Read the model definition and answer for the solid it produces. Units are mm, in the model's axes. Face numbers are marked on the shaded views. A direction names the side the tool comes from. Coordinates: 2 decimals unless noted, no trailing zeros. Write each loop counter-clockwise with the first axis right and the second up, starting at its lowest first coordinate (ties: lowest second). Pieces come first, ordered by that corner, then holes. Notation, with made-up numbers: (-5.5, -6) -> (41.5, -6) arc R10 ccw to (41.5, 13) -> close; hole circle Ø10 at (21, -19). An arc over 180 degrees is marked (long way). Use CSV: the item, a comma, the result in double quotes.
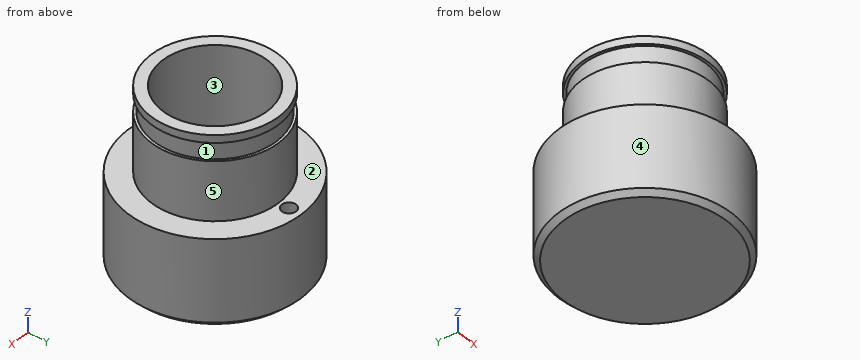
from build123d import *

# Parameters (mm, degrees)
ESQUISSE1_R                    = 17
BOSS_EXTRU_1_DEPTH             = 17
ESQUISSE2_R                    = 12.5
BOSS_EXTRU_2_DEPTH             = 11.5
ESQUISSE3_R                    = 12
BOSS_EXTRU_3_DEPTH             = 3.5
ESQUISSE4_R                    = 12.5
BOSS_EXTRU_4_DEPTH             = 1.5
ESQUISSE5_R                    = 10.25
ENL_V_MAT_EXTRU_1_DEPTH        = 30
ESQUISSE6_R                    = 10.25
ESQUISSE6_R_2                  = 6.75
ENL_V_MAT_EXTRU_2_DEPTH        = 1.5
ESQUISSE7_R                    = 12
ESQUISSE7_R_2                  = 10.25
ENL_V_MAT_EXTRU_3_DEPTH        = 2
F_2_8_2_8_DIAMETER_HOLE1_D     = 2.8
F_2_8_2_8_DIAMETER_HOLE1_DEPTH = 12
F_2_8_2_8_DIAMETER_HOLE1_TIP   = 0.841204867
CHANFREIN1_SIZE                = 1


with BuildPart() as part:
    # Esquisse1 → Boss.-Extru.1 (new body)
    with BuildSketch(Plane.XY):
        Circle(ESQUISSE1_R)
    extrude(amount=BOSS_EXTRU_1_DEPTH)

    # Esquisse2 → Boss.-Extru.2 (add)
    with BuildSketch(Plane.XY.offset(17)):
        Circle(ESQUISSE2_R)
    extrude(amount=BOSS_EXTRU_2_DEPTH)

    # Esquisse3 → Boss.-Extru.3 (add)
    with BuildSketch(Plane.XY.offset(28.5)):
        Circle(ESQUISSE3_R)
    extrude(amount=BOSS_EXTRU_3_DEPTH)

    # Esquisse4 → Boss.-Extru.4 (add)
    with BuildSketch(Plane.XY.offset(32)):
        Circle(ESQUISSE4_R)
    extrude(amount=BOSS_EXTRU_4_DEPTH)

    # Esquisse5 → Enlèv. mat.-Extru.1 (cut)
    with BuildSketch(Plane.XY.offset(33.5)):
        Circle(ESQUISSE5_R)
    extrude(amount=-ENL_V_MAT_EXTRU_1_DEPTH, mode=Mode.SUBTRACT)

    # Esquisse6 → Enlèv. mat.-Extru.2 (cut)
    with BuildSketch(Plane.XY.offset(3.5)):
        Circle(ESQUISSE6_R)
        Circle(ESQUISSE6_R_2, mode=Mode.SUBTRACT)
    extrude(amount=-ENL_V_MAT_EXTRU_2_DEPTH, mode=Mode.SUBTRACT)

    # Esquisse7 → Enlèv. mat.-Extru.3 (cut)
    with BuildSketch(Plane.XY.offset(3.5)):
        Circle(ESQUISSE7_R)
        Circle(ESQUISSE7_R_2, mode=Mode.SUBTRACT)
    extrude(amount=ENL_V_MAT_EXTRU_3_DEPTH, mode=Mode.SUBTRACT)

    # Ø2.8 (2.8) Diameter Hole1
    with Locations(Plane.XY.offset(17)):
        with Locations((0, 14.5)):
            Hole(F_2_8_2_8_DIAMETER_HOLE1_D / 2, depth=F_2_8_2_8_DIAMETER_HOLE1_DEPTH)
            with Locations((0, 0, -(F_2_8_2_8_DIAMETER_HOLE1_DEPTH + F_2_8_2_8_DIAMETER_HOLE1_TIP / 2))):  # 118° drill point
                Cone(0, F_2_8_2_8_DIAMETER_HOLE1_D / 2, F_2_8_2_8_DIAMETER_HOLE1_TIP, mode=Mode.SUBTRACT)

    # Chanfrein1
    chanfrein1_edges = [part.edges().sort_by_distance(p)[0] for p in [
        (-17, 0, 0),
    ]]
    chamfer(chanfrein1_edges, length=CHANFREIN1_SIZE)


solid = part.part
1. For a pull along Y with two mould halves and no side action, classify the marked faces 1, 2 and 3 as pulls with the +Y half, pulls with the -Y half, needs draft (parallel to the pull), parting line crosses it, or undercut.
Solutions:
face 1,"parting line crosses it"
face 2,"needs draft"
face 3,"undercut"
2. A cutting plane is placed at A-A (z = 10). Give the vertices of the cut face in (x, y), and give its area (3 significant figures).
Solutions:
outline,"circle Ø34 at (0, 0); hole circle Ø20.5 at (0, 0); hole circle Ø2.8 at (0, 14.5)"
area,"572 mm^2"
3. Find the intervals of material crossed by line 1 along Y through (x, z) = (0, 3.2); line 2 along Y through (x, z) = (0, 10); line 3 along Y through (x, z) = (0, 19.5), in increasing order.
Solutions:
line 1,"y = -17 to -10.25, -6.75 to 6.75, 10.25 to 17"
line 2,"y = -17 to -10.25, 10.25 to 13.1, 15.9 to 17"
line 3,"y = -12.5 to -10.25, 10.25 to 12.5"
4. A tool of negligible diameter and unlimited length cuts with its end or side. For the marked faces 4 and 5, from which of +Z, -Z, +X, -X, +Y, -Y can it reach the whole face along a straight path? Write none if from no direction.
Solutions:
face 4,"+Z, -Z"
face 5,"+Z"
5. A cutting plane is placed at B-B (z = 21). Give the vertices of the cut face in (x, y), and give its area (3 significant figures).
Solutions:
outline,"circle Ø25 at (0, 0); hole circle Ø20.5 at (0, 0)"
area,"161 mm^2"
6. Each of these flat-tipped pins is pushed along its axis until it touches: pin 1 Ø7.5 at (x, y) = (-3, -3.5) entering from +Z; pin 2 Ø6 at (y, z) = (-8.5, 13) entering from +X; pin 3 Ø5 at (y, z) = (-6, 12.5) entering from -X. Where does it stop, or does it pass through?
Solutions:
pin 1,"stops at z = 3.5"
pin 2,"stops at x = 16.09"
pin 3,"stops at x = -16.64"
